from build123d import *

# Parameters (mm, degrees)
SKETCH1_R           = 12
SKETCH1_R_2         = 7.5
BOSS_EXTRUDE1_DEPTH = 14
SKETCH1_5_R         = 17.5
SKETCH1_5_R_2       = 12
BOSS_EXTRUDE3_DEPTH = 21
BOSS_EXTRUDE4_DEPTH = 9
CUT_EXTRUDE3_START  = 2.5
CUT_EXTRUDE3_DEPTH  = 6.5
FILLET1_R           = 24


with BuildPart() as part:
    # Sketch1 → Boss-Extrude1 (new body, symmetric)
    with BuildSketch(Plane.XY):
        Circle(SKETCH1_R)
        Circle(SKETCH1_R_2, mode=Mode.SUBTRACT)
    extrude(amount=BOSS_EXTRUDE1_DEPTH, both=True)



with BuildPart() as body_2:
    # Sketch1<5> → Boss-Extrude3 (new body, symmetric)
    with BuildSketch(Plane.XY):
        with Locations((177.137212096, 0)):
            Circle(SKETCH1_5_R)
        with Locations((177.137212096, 0)):
            Circle(SKETCH1_5_R_2, mode=Mode.SUBTRACT)
    extrude(amount=BOSS_EXTRUDE3_DEPTH, both=True)


with BuildPart() as part_1:
    add(part.part)

    add(body_2.part)  # Boss-Extrude4 merges body 2
    # Sketch1<6> → Boss-Extrude4 (add, symmetric)
    with BuildSketch(Plane.XY):
        with BuildLine():
            Line((162.128881076, 9), (7.937253933, 9))
            ThreePointArc((7.937253933, 9), (10.937253933, 4.937253933), (12, 0))
            ThreePointArc((12, 0), (10.937253933, -4.937253933), (7.937253933, -9))
            Line((7.937253933, -9), (162.128881076, -9))
            ThreePointArc((162.128881076, -9), (159.637212096, 0), (162.128881076, 9))
        make_face()
    extrude(amount=BOSS_EXTRUDE4_DEPTH, both=True)

    # Sketch2 → Cut-Extrude3 (cut)
    with BuildSketch(Plane.XY.offset(CUT_EXTRUDE3_START)):
        with BuildLine():
            Line((21, 5), (151, 5))
            ThreePointArc((151, 5), (156, 0), (151, -5))
            Line((151, -5), (21, -5))
            ThreePointArc((21, -5), (16, 0), (21, 5))
        make_face()
    cut_extrude3 = extrude(amount=CUT_EXTRUDE3_DEPTH, mode=Mode.SUBTRACT)

    # Mirror1: Cut-Extrude3 across plane
    add(cut_extrude3.mirror(Plane.XY), mode=Mode.SUBTRACT)

    # Fillet1
    fillet1_edges = [part_1.edges().sort_by_distance(p)[0] for p in [
        (7.937253933, 9, 0),
        (7.937253933, -9, 0),
        (162.128881076, -9, 0),
        (162.128881076, 9, 0),
    ]]
    fillet(fillet1_edges, radius=FILLET1_R)


solid = part_1.part
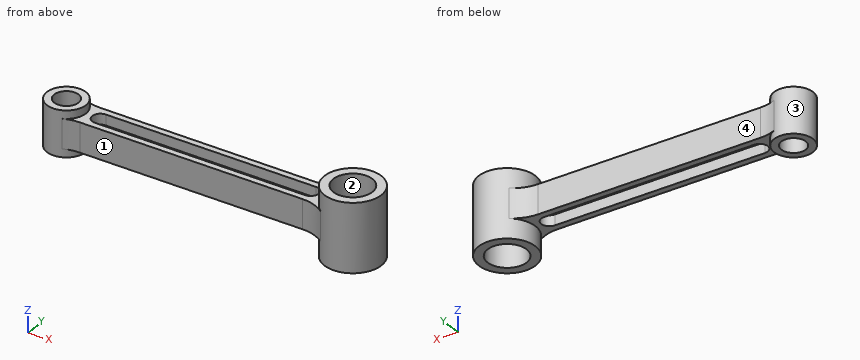
Geometry check sheet. Reference: the model listing, model coordinates, mm. Face numbers are marked on the shaded views. A direction names the side the tool comes from. Round coordinates to 2 decimals unless told otherwise and drop trailing zeros. Loops run counter-clockwise (first coordinate to the right, second up) from the corner with the lowest first, then second, coordinate; pieces in that order, holes last.
Item 1: Cross-section at B-B on x = 0. Record the boundary of the cut face in (y, z).
Item 2: Gauge pin test, flat ends, axial feed: pin 1 (3 mm diameter, centred on x = 118, z = -6, fed in from -Y); pin 2 (7 mm diameter, centred on x = -3.5, y = -2.5, fed in from -Z); pin 3 (5 mm diameter, centred on x = 71, y = 0.5, fed in from +Z). Record the tip position at first contact, or that the pin passes through.
Item 3: Cross-section at C-C on z = -7. Record the boundary of the cut face in (x, y).
Item 4: Thickness scan on line 1 (Y direction, x = 126.5, z = -3); line 2 (X direction, y = -4.5, z = -3); line 3 (Y direction, x = 0, z = 0.75). Record the ranges inside material, lowest first.
Item 5: Access from +Z, -Z, +X, -X, +Y, -Y to the whole of each face (thin tool, end or side, straight path). Record for the marked faces 1, 2, 3 and 4.
Item 6: Cross-section at D-D on x = 132. Record the boundary of the cut face in (y, z), then the cut area to 3 significant figures.
Item 7: Cross-section at A-A on y = 0. Record the boundary of the cut face in (x, z), then the cut area to 3 significant figures.
Answer sheet:
1. outline: (-12, -14) - (-7.5, -14) - (-7.5, 14) - (-12, 14) - close; (7.5, -14) - (12, -14) - (12, 14) - (7.5, 14) - close
2. pin 1: stops at y = -9
2. pin 2: stops at z = -14
2. pin 3: stops at z = 2.5
3. outline: (4.8, -11) arc R24 cw to (14.39, -9) - (151.97, -9) arc R24 cw to (166.53, -13.92) arc R17.5 ccw (long way) to (166.53, 13.92) arc R24 cw to (151.97, 9) - (14.39, 9) arc R24 cw to (4.8, 11) arc R12 ccw (long way) to start; hole circle Ø15 at (0, 0); hole (21, -5) - (151, -5) arc R5 ccw to (151, 5) - (21, 5) arc R5 ccw to start; hole circle Ø24 at (177.14, 0)
4. line 1: y = -9 to -5, 5 to 9
4. line 2: x = -11.12 to -6, 6 to 18.82, 153.18 to 166.01, 188.26 to 194.05
4. line 3: y = -12 to -7.5, 7.5 to 12
5. face 1: +Z, -Z, -Y
5. face 2: +Z, -Z
5. face 3: none
5. face 4: +Z, -Z, +Y
6. outline: (-9, -9) - (-5, -9) - (-5, -2.5) - (5, -2.5) - (5, -9) - (9, -9) - (9, 9) - (5, 9) - (5, 2.5) - (-5, 2.5) - (-5, 9) - (-9, 9) - close
6. area: 194 mm2
7. outline: (-12, -14) - (-7.5, -14) - (-7.5, 14) - (-12, 14) - close; (7.5, -14) - (12, -14) - (12, -9) - (16, -9) - (16, -2.5) - (156, -2.5) - (156, -9) - (159.64, -9) - (159.64, -21) - (165.14, -21) - (165.14, 21) - (159.64, 21) - (159.64, 9) - (156, 9) - (156, 2.5) - (16, 2.5) - (16, 9) - (12, 9) - (12, 14) - (7.5, 14) - close; (189.14, -21) - (194.64, -21) - (194.64, 21) - (189.14, 21) - close
7. area: 1,550 mm2
